Here's how the part is built. I have some questions about the finished solid (model axes, mm). Face numbers are marked on the shaded views. A direction names the side the tool comes from. Give positions to 0.01 mm unless a question says otherwise; leave off trailing zeros. Loops run counter-clockwise (first coordinate to the right, second up) from the corner with the lowest first, then second, coordinate; pieces in that order, holes last. Notation, with made-up numbers: (39, 0) - (56, 0) arc R24 ccw to (56, 37) - close; hole circle Ø3 at (2, 4). An arc over 180 degrees is marked (long way). Use a Markdown table: item, result.
from build123d import *

# Parameters (mm, degrees)
PAD_DEPTH = 5


with BuildPart() as part:
    # Sketch → Pad (new body, symmetric)
    with BuildSketch(Plane.YZ):
        with BuildLine():
            ThreePointArc((-1.299038, -0.75), (1.5, 0), (-1.299038, 0.75))
            Line((-1.299038, 0.75), (-7.5, 0.75))
            Line((-7.5, 0.75), (-11.5, 3))
            Line((-11.5, 3), (3.5, 3))
            Line((3.5, -3), (3.5, 3))
            Line((-11.5, -3), (3.5, -3))
            Line((-7.5, -0.75), (-11.5, -3))
            Line((-1.299038, -0.75), (-7.5, -0.75))
        make_face()
    extrude(amount=PAD_DEPTH, both=True)


solid = part.part
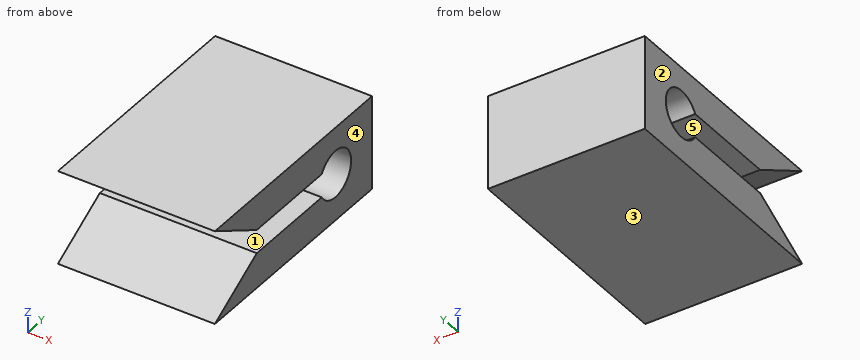
(1) Suppose I cut it at C-C on y = -3. Write out the boundary of the cut face in (x, z).
A:
| item | result |
|---|---|
| outline | (-5, -3) - (5, -3) - (5, -0.75) - (-5, -0.75) - close; (-5, 0.75) - (5, 0.75) - (5, 3) - (-5, 3) - close |
(2) Suppose I cut it at B-B on x = 2.75. Write out the boundary of the cut face in (y, z), plus the area to 3 significant figures.
A:
| item | result |
|---|---|
| outline | (-11.5, -3) - (3.5, -3) - (3.5, 3) - (-11.5, 3) - (-7.5, 0.75) - (-1.3, 0.75) arc R1.5 cw (long way) to (-1.3, -0.75) - (-7.5, -0.75) - close |
| area | 58.8 mm2 |
(3) If I drill on line 1 (Z direction, x = -0.5, y = -2.75); line 2 (Y direction, x = 1, z = 0), over which ranges is the centre line in solid material (lowest first)?
A:
| item | result |
|---|---|
| line 1 | -3 to -0.75, 0.75 to 3 |
| line 2 | 1.5 to 3.5 |
(4) We'd pull the mould along Z, two halves only. Please class the marked faces 3, 4 and 5: pulls with the +Z half, pulls with the -Z half, needs draft (parallel to the pull), parting line crosses it, or undercut.
A:
| item | result |
|---|---|
| face 3 | pulls with the -Z half |
| face 4 | needs draft |
| face 5 | undercut |
(5) Suppose I cut it at A-A on y = 0. Write out the boundary of the cut face in (x, z), plus the area to 3 significant figures.
A:
| item | result |
|---|---|
| outline | (-5, -3) - (5, -3) - (5, -1.5) - (-5, -1.5) - close; (-5, 1.5) - (5, 1.5) - (5, 3) - (-5, 3) - close |
| area | 30.0 mm2 |
(6) Will these pins go through, and if not, where does the flat tip stop? pin 1 (1.5 mm diameter, centred on x = 1.5, z = 2, fed in from -Y); pin 2 (3.5 mm diameter, centred on y = 0, z = 0, fed in from -X).
A:
| item | result |
|---|---|
| pin 1 | y = -11.06 |
| pin 2 | x = -5 |
(7) Suppose I cut it at D-D on z = 0. Write out the boundary of the cut face in (x, y).
A:
| item | result |
|---|---|
| outline | (-5, 1.5) - (5, 1.5) - (5, 3.5) - (-5, 3.5) - close |
(8) On a 3-axis mill with a long thin cutter (end or side, diameter ignored), from which of +Z, -Z, +X, -X, +Y, -Y can I reach the whole of each face in a straight line? I mean the marked faces 1 and 2. Say none if no direction works.
A:
| item | result |
|---|---|
| face 1 | +X, -X, -Y |
| face 2 | +Z, -Z, -X, +Y, -Y |
